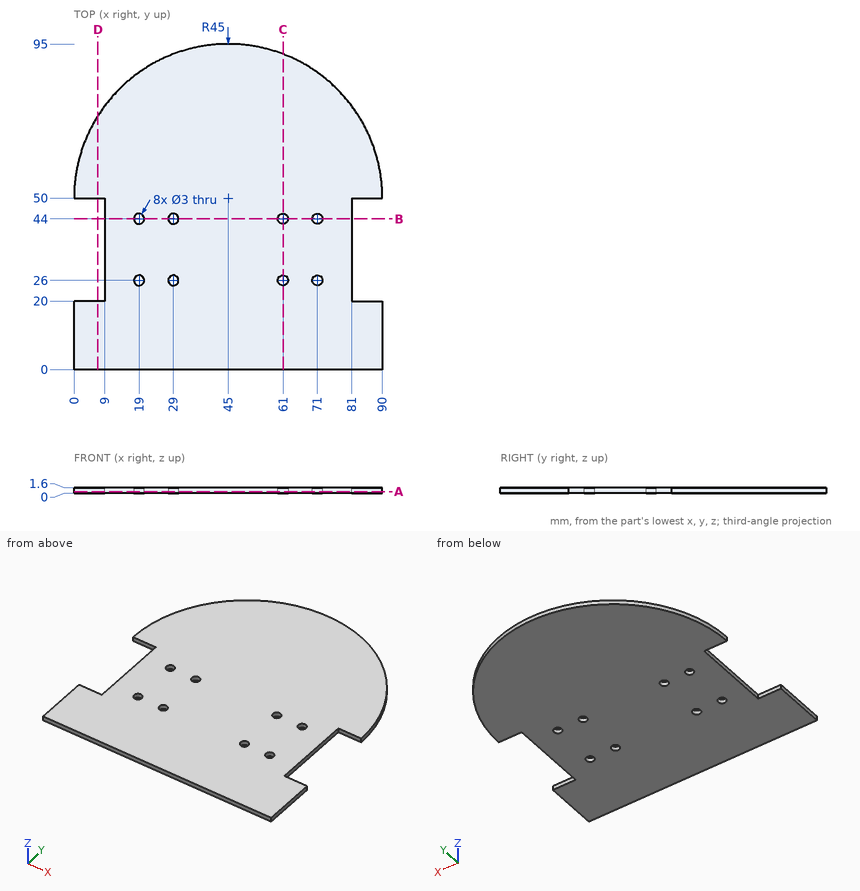
Part print with two shaded views. Sizes in mm from the minimum x, y, z corner. Round coordinates to 2 decimals unless told otherwise and drop trailing zeros. Order: outer loops, then holes, each group sorted by start corner. A loop starts at its lowest first (then second) coordinate and runs counter-clockwise, first axis right, second up. Notation, with made-up numbers: (10, 34.5) - (59, 34.5) arc R6 ccw to (59, 44.5) - close; hole circle Ø4 at (71, -33). An arc over 180 degrees is marked (long way). Answer in a Markdown table with one row per item. Add a question column.
(1) Probe L1, parallel to X at y = 44, z = 0.35; L2, parallel to Y at x = 71, z = 0.65; L3, parallel to Y at x = 4.5, z = 1.4. List the from-to ranges inside material, lowest first. Write a range as [from, to].
(2) Drop a flat-ended pin along its axis: pin 1 Ø0.8 at (x, z) = (83.5, 1) entering from +Y. Give the stop position or say it passes through.
(3) Band-saw the part on D-D on x = 7. List the corners of the cut face in (y, z).
(4) Band-saw the part on A-A on z = 0.4. Count the separate pieces of the cut face and the enclosed holes in it, and give its area (3 significant figures).
(5) Band-saw the part on C-C on x = 61. List the corners of the cut face in (y, z), and give its area (3 significant figures).
(6) Band-saw the part on B-B on y = 44. List the corners of the cut face in (x, z).
Data:
| question | item | result |
|---|---|---|
| 1 | L1 | x = [9, 17.5], [20.5, 27.5], [30.5, 59.5], [62.5, 69.5], [72.5, 81] |
| 1 | L2 | y = [0, 24.5], [27.5, 42.5], [45.5, 86.73] |
| 1 | L3 | y = [0, 20], [50, 69.62] |
| 2 | pin 1 | stops at y = 73.95 |
| 3 | outline | (0, 0) - (20, 0) - (20, 1.6) - (0, 1.6) - close; (50, 0) - (74.1, 0) - (74.1, 1.6) - (50, 1.6) - close |
| 4 | separate pieces | 1 |
| 4 | enclosed holes | 8 |
| 4 | area | 7,080 mm^2 |
| 5 | outline | (0, 0) - (24.5, 0) - (24.5, 1.6) - (0, 1.6) - close; (27.5, 0) - (42.5, 0) - (42.5, 1.6) - (27.5, 1.6) - close; (45.5, 0) - (92.06, 0) - (92.06, 1.6) - (45.5, 1.6) - close |
| 5 | area | 138 mm^2 |
| 6 | outline | (9, 0) - (17.5, 0) - (17.5, 1.6) - (9, 1.6) - close; (20.5, 0) - (27.5, 0) - (27.5, 1.6) - (20.5, 1.6) - close; (30.5, 0) - (59.5, 0) - (59.5, 1.6) - (30.5, 1.6) - close; (62.5, 0) - (69.5, 0) - (69.5, 1.6) - (62.5, 1.6) - close; (72.5, 0) - (81, 0) - (81, 1.6) - (72.5, 1.6) - close |
